Build history of the part. All positions in model axes, mm. A direction names the side the tool comes from. Give positions to 0.01 mm unless a question says otherwise; leave off trailing zeros. Loops run counter-clockwise (first coordinate to the right, second up) from the corner with the lowest first, then second, coordinate; pieces in that order, holes last. Notation, with made-up numbers: (75.5, -15) -> (87.5, -15) arc R28 ccw to (87.5, 20) -> close; hole circle Ø10 at (7, -36.75). An arc over 180 degrees is marked (long way). Answer as a JSON object with one key per item and string values. Group by question number.
from build123d import *

# Parameters (mm, degrees)
SKETCH1_R                                           = 11
BOSS_EXTRUDE1_DEPTH                                 = 20
SKETCH2_R                                           = 21
CUT_EXTRUDE1_DEPTH                                  = 15
CBORE_FOR_M4_HEX_SOCKET_HEAD_CAP_SCREW2_D           = 4.5
CBORE_FOR_M4_HEX_SOCKET_HEAD_CAP_SCREW2_CBORE_D     = 8
CBORE_FOR_M4_HEX_SOCKET_HEAD_CAP_SCREW2_CBORE_DEPTH = 4.4
CUT_EXTRUDE2_REACH                                  = 57.743
SKETCH5_R                                           = 1.65
FILLET1_R                                           = 2.5


with BuildPart() as part:
    # Sketch1 → Boss-Extrude1 (new body)
    with BuildSketch(Plane(origin=(0, 0, 0), x_dir=(1, 0, 0), z_dir=(0, 1, 0))):
        Polygon((-25, -25), (-38.5, -25), (-38.5, -35), (38.5, -35), (38.5, -25), (25, -25), (25, 25), (-25, 25), align=None)
        with Locations(Location((0, 0, 0), (0, 0, 270))):
            Circle(SKETCH1_R, mode=Mode.SUBTRACT)
    extrude(amount=BOSS_EXTRUDE1_DEPTH)

    # Sketch2 → Cut-Extrude1 (cut)
    with BuildSketch(Plane(origin=(0, 20, 0), x_dir=(1, 0, 0), z_dir=(0, 1, 0))):
        with Locations(Location((0, 0, 0), (0, 0, 270))):
            Circle(SKETCH2_R)
    extrude(amount=-CUT_EXTRUDE1_DEPTH, mode=Mode.SUBTRACT)

    # CBORE for M4 Hex Socket Head Cap Screw2 (through all)
    with Locations(Plane(origin=(31.75, 10, 25), x_dir=(-1, 0, 0), z_dir=(0, 0, -1))):
        with Locations((0, 0), (63.5, 0)):
            CounterBoreHole(CBORE_FOR_M4_HEX_SOCKET_HEAD_CAP_SCREW2_D / 2, CBORE_FOR_M4_HEX_SOCKET_HEAD_CAP_SCREW2_CBORE_D / 2, CBORE_FOR_M4_HEX_SOCKET_HEAD_CAP_SCREW2_CBORE_DEPTH)

    # Sketch5 → Cut-Extrude2 (cut, up to next)
    with BuildSketch(Plane.XZ, mode=Mode.PRIVATE) as cut_extrude2_sk1:
        with Locations(Location((12.990381057, 7.5, 0), (0, 0, 270))):
            Circle(SKETCH5_R)
    cut_extrude2_tool1 = extrude(cut_extrude2_sk1.sketch, amount=-CUT_EXTRUDE2_REACH, mode=Mode.PRIVATE) & part.part
    # Sketch5 → Cut-Extrude2 (cut, up to next)
    with BuildSketch(Plane.XZ, mode=Mode.PRIVATE) as cut_extrude2_sk2:
        with Locations(Location((-12.990381057, 7.5, 0), (0, 0, 270))):
            Circle(SKETCH5_R)
    cut_extrude2_tool2 = extrude(cut_extrude2_sk2.sketch, amount=-CUT_EXTRUDE2_REACH, mode=Mode.PRIVATE) & part.part
    # Sketch5 → Cut-Extrude2 (cut, up to next)
    with BuildSketch(Plane.XZ, mode=Mode.PRIVATE) as cut_extrude2_sk3:
        with Locations(Location((0, -15, 0), (0, 0, 270))):
            Circle(SKETCH5_R)
    cut_extrude2_tool3 = extrude(cut_extrude2_sk3.sketch, amount=-CUT_EXTRUDE2_REACH, mode=Mode.PRIVATE) & part.part
    add(cut_extrude2_tool1.solids().sort_by_distance((12.990381, 0, 7.5))[0], mode=Mode.SUBTRACT)
    add(cut_extrude2_tool2.solids().sort_by_distance((-12.990381, 0, 7.5))[0], mode=Mode.SUBTRACT)
    add(cut_extrude2_tool3.solids().sort_by_distance((0, 0, -15))[0], mode=Mode.SUBTRACT)

    # Fillet1
    fillet1_edges = [part.edges().sort_by_distance(p)[0] for p in [
        (-31.75, 0, 25),
        (-25, 0, 0),
        (0, 0, -25),
        (-31.75, 20, 25),
        (25, 10, -25),
        (25, 10, 25),
        (-25, 10, 25),
        (-25, 10, -25),
        (31.75, 20, 25),
        (25, 20, 0),
        (0, 20, -25),
        (25, 0, 0),
        (-25, 20, 0),
        (31.75, 0, 25),
    ]]
    fillet(fillet1_edges, radius=FILLET1_R)


solid = part.part
(1) Saw through at C-C on x = 0. List the corners of the cut face in (y, z), plus the area to 3 significant figures.
(2) Saw through at B-B on z = 0. List the corners of the cut face in (x, y).
(3) Saw through at D-D on z = 7.5. List the corners of the cut face in (x, y), plus the area to 3 significant figures.
(4) Probe line 1 along X through (y, z) = (3.25, 0); line 2 along Y through (x, z) = (-31.75, 28.35); line 3 along X through (y, z) = (2.05, 7.5). List the from-to ranges inside material, lowest first. Write a range as [from, to].
(5) Pull direction Z, two halves, no side cores. Call faces 1 (the cylindrical face through (-10.74, 2.46, -2.38)), 2 (the flat face through (-38.5, 10, 30)), 3 (the flat face through (-1, 10, 35)): pulls with the +Z half, pulls with the -Z half, needs draft (parallel to the pull), parting line crosses it, or undercut.
(6) 3-axis set-ups, long thin cutter, end or side, ignore diameter. For faces 4 (the cylindrical face through (-24.287, 19.248, 0.315)), 5 (the cylindrical face through (24.248, 19.287, -0.315)), 6 (the flat face through (-9, 5, 9)): which of +Z, -Z, +X, -X, +Y, -Y reach the whole face in a straight line?
(7) Saw through at A-A on x = -31.75. List the corners of the cut face in (y, z).
(8) Pin check, flat tips, straight feed: pin 1 (3 mm diameter, centred on x = -12.99, z = 7.5, fed in from -Y); pin 2 (9 mm diameter, centred on x = -32, y = 11, fed in from -Z); pin 3 (2 mm diameter, centred on x = 24.5, z = -1, fed in from +Y); pin 4 (2.5 mm diameter, centred on x = -30.5, y = 10.5, fed in from -Z). Stop position of each tip, or through.
Calculated:
{
 "1": {"outline": "(0, -22.5) arc R2.5 ccw to (2.5, -25) -> (17.5, -25) arc R2.5 ccw to (20, -22.5) -> (20, -21) -> (5, -21) -> (5, -16.65) -> (0, -16.65) -> close; (0, -13.35) -> (5, -13.35) -> (5, -11) -> (0, -11) -> close; (0, 11) -> (5, 11) -> (5, 21) -> (20, 21) -> (20, 35) -> (0, 35) -> close", "area": "441 mm^2"},
 "2": {"outline": "(-25, 2.5) arc R2.5 ccw to (-22.5, 0) -> (-11, 0) -> (-11, 5) -> (-21, 5) -> (-21, 20) -> (-22.5, 20) arc R2.5 ccw to (-25, 17.5) -> close; (11, 0) -> (22.5, 0) arc R2.5 ccw to (25, 2.5) -> (25, 17.5) arc R2.5 ccw to (22.5, 20) -> (21, 20) -> (21, 5) -> (11, 5) -> close"},
 "3": {"outline": "(-25, 2.5) arc R2.5 ccw to (-22.5, 0) -> (-14.64, 0) -> (-14.64, 5) -> (-19.62, 5) -> (-19.62, 20) -> (-22.5, 20) arc R2.5 ccw to (-25, 17.5) -> close; (-11.34, 0) -> (-8.05, 0) -> (-8.05, 5) -> (-11.34, 5) -> close; (8.05, 0) -> (11.34, 0) -> (11.34, 5) -> (8.05, 5) -> close; (14.64, 0) -> (22.5, 0) arc R2.5 ccw to (25, 2.5) -> (25, 17.5) arc R2.5 ccw to (22.5, 20) -> (19.62, 20) -> (19.62, 5) -> (14.64, 5) -> close", "area": "293 mm^2"},
 "4": {"line 1": "x = [-25, -11], [11, 25]", "line 2": "y = [0, 6], [14, 20]", "line 3": "x = [-24.96, -14.64], [-11.34, -8.05], [8.05, 11.34], [14.64, 24.96]"},
 "5": {"face 1": "undercut", "face 2": "needs draft", "face 3": "pulls with the +Z half"},
 "6": {"face 4": "-Z, -X, +Y", "face 5": "-Z, +X, +Y", "face 6": "+Y"},
 "7": {"outline": "(0, 27.5) arc R2.5 ccw to (2.5, 25) -> (6, 25) -> (6, 29.4) -> (7.75, 29.4) -> (7.75, 35) -> (0, 35) -> close; (12.25, 29.4) -> (14, 29.4) -> (14, 25) -> (17.5, 25) arc R2.5 ccw to (20, 27.5) -> (20, 35) -> (12.25, 35) -> close"},
 "8": {"pin 1": "passes through", "pin 2": "stops at z = 25", "pin 3": "stops at y = 19.79", "pin 4": "stops at z = 29.4"}
}
